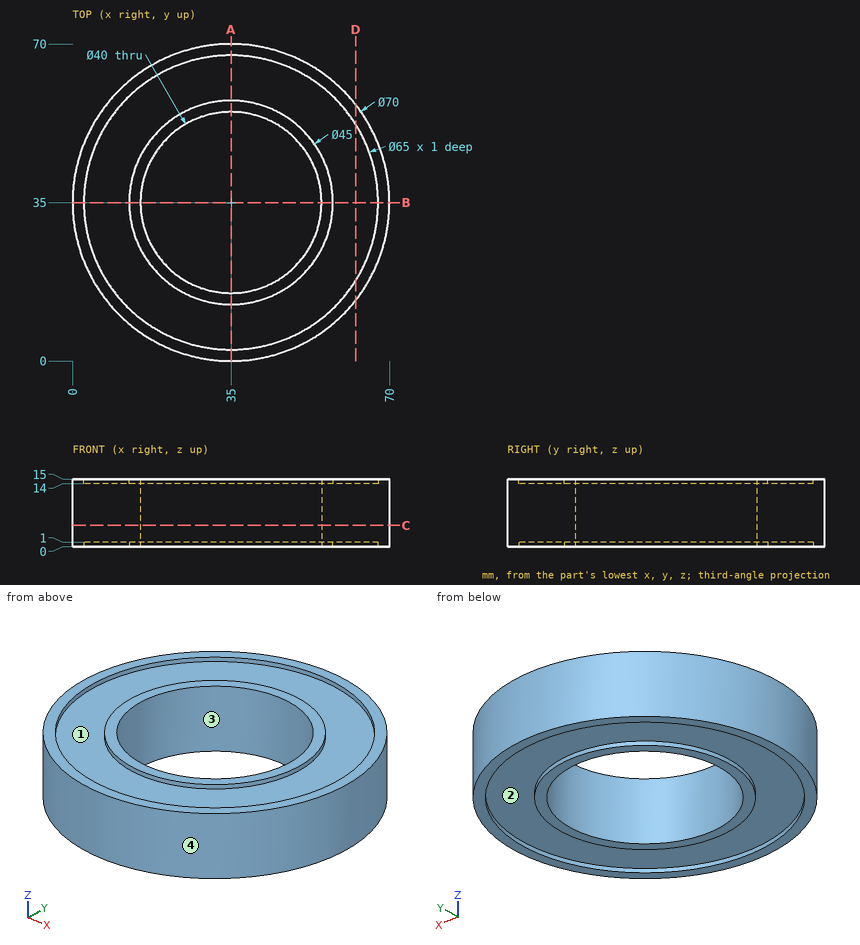
Verification items for this drawing (mm, ordinates from the low corner). A direction names the side the tool comes from. Coordinates: 2 decimals unless noted, no trailing zeros. Write each loop counter-clockwise with the first axis right and the second up, starting at its lowest first coordinate (ties: lowest second). Pieces come first, ordered by that corner, then holes. Notation, with made-up numbers: M 72.5,-29 L 110.5,-29 A26 ccw 110.5,5 Z; hole C 18,37.25 d4. An arc over 180 degrees is marked long. Use CSV: the item, a comma, the result in double quotes.
Q1. Go/stop test with flat-tipped pins: P1, Ø1, axis at y = 12.5, z = 3.5, coming from the -X side; P2, Ø24, axis at x = 35, y = 35, coming from the -Z side; P3, Ø4, axis at y = 22.5, z = 9.5, coming from the +X side; P4, Ø1.5, axis at y = 13, z = 8, coming from the +X side. Record where each tip stops, or that it passes through.
Computed values:
P1,"x = 7.78"
P2,"through"
P3,"x = 68.39"
P4,"x = 62.81"
Q2. Section check A-A, the plane x = 35. Enter the section's corners in (y, z), and give its area (3 significant figures).
Computed values:
outline,"M 0,0 L 2.5,0 L 2.5,1 L 12.5,1 L 12.5,0 L 15,0 L 15,15 L 12.5,15 L 12.5,14 L 2.5,14 L 2.5,15 L 0,15 Z; M 55,0 L 57.5,0 L 57.5,1 L 67.5,1 L 67.5,0 L 70,0 L 70,15 L 67.5,15 L 67.5,14 L 57.5,14 L 57.5,15 L 55,15 Z"
area,"410 mm²"
Q3. Section check D-D, the plane x = 62.5. Enter the section's corners in (y, z), and give its area (3 significant figures).
Computed values:
outline,"M 13.35,0 L 17.68,0 L 17.68,1 L 52.32,1 L 52.32,0 L 56.65,0 L 56.65,15 L 52.32,15 L 52.32,14 L 17.68,14 L 17.68,15 L 13.35,15 Z"
area,"580 mm²"
Q4. Mould release check, pull along Y, two halves, no side actions. Record for the marked faces 3 and 4: pulls with the +Y half, pulls with the -Y half, needs draft (parallel to the pull), parting line crosses it, or undercut.
Computed values:
face 3,"undercut"
face 4,"parting line crosses it"
Q5. Set-up check for the marked faces 1 and 2: record each of +Z, -Z, +X, -X, +Y, -Y from which the full face is reachable in a straight line by a thin tool's end or side.
Computed values:
face 1,"+Z"
face 2,"-Z"
Q6. Section check C-C, the plane z = 4.75. Enter the section's corners in (x, y).
Computed values:
outline,"C 35,35 d70; hole C 35,35 d40"
Q7. Thickness scan on line 1 along Z through (x, y) = (39, 58); line 2 along Y through (x, z) = (38, 12); line 3 along Y through (x, z) = (18.5, 7). Record the ranges inside material, lowest first. Write a range as [from, to].
Computed values:
line 1,"[1, 14]"
line 2,"[0.13, 15.23], [54.77, 69.87]"
line 3,"[4.13, 23.7], [46.3, 65.87]"
